Model file for the job. Use its own axes, mm. A direction names the side the tool comes from. Coordinates: 2 decimals unless noted, no trailing zeros. Write each loop counter-clockwise with the first axis right and the second up, starting at its lowest first coordinate (ties: lowest second). Pieces come first, ordered by that corner, then holes. Notation, with made-up numbers: M 60,-21 L 71,-21 A16 cw 71,-13 Z; hole C -29.5,8 d11. An arc over 180 degrees is marked long. Put each result on its own line as item: value. Start each with the question number.
Q1. Drop a flat-ended pin along its axis: pin 1 (1.5 mm diameter, centred on x = 5.5, z = -27, fed in from +Y). Give the stop position or say it passes through.
Q2. Which spindle directions (+Z, -Z, +X, -X, +Y, -Y) get a long thin tool onto all of the face, cutting with end or side? Do faces 1 (the flat face through (-2, 0, -1)), 2 (the flat face through (-2, 14.5, -27)). Say none if no direction does.
Q3. Cut at A-A (x = 2.5). Write the cut outline in (y, z).
Q4. Drill centre lines: line 1 along Z through (x, y) = (20, 15.25); line 2 along Z through (x, y) = (14, 14.75). Where is each one in solid material? Low to high.
```python
from build123d import *

# Parameters (mm, degrees)
SKETCH1_W           = 54
SKETCH1_H           = 60
BOSS_EXTRUDE1_DEPTH = 17
SKETCH2_W           = 54
SKETCH2_H           = 6
CUT_EXTRUDE1_DEPTH  = 2.5
FILLET1_R           = 1


with BuildPart() as part:
    # Sketch1 → Boss-Extrude1 (new body)
    with BuildSketch(Plane(origin=(0, 0, 0), x_dir=(1, 0, 0), z_dir=(0, 1, 0))):
        with Locations((-2.044526592, -0.229360244)):
            Rectangle(SKETCH1_W, SKETCH1_H)
    extrude(amount=BOSS_EXTRUDE1_DEPTH)

    # Sketch2 → Cut-Extrude1 (cut)
    with BuildSketch(Plane(origin=(0, 17, 0), x_dir=(1, 0, 0), z_dir=(0, 1, 0))):
        with Locations((-2.044526592, 26.770639756)):
            Rectangle(SKETCH2_W, SKETCH2_H)
    extrude(amount=-CUT_EXTRUDE1_DEPTH, mode=Mode.SUBTRACT)

    # Fillet1
    fillet1_edges = [part.edges().sort_by_distance(p)[0] for p in [
        (24.955473408, 17, 3.229360244),
        (-29.044526592, 17, 3.229360244),
        (-29.044526592, 14.5, -26.770639756),
        (-29.044526592, 15.75, -23.770639756),
        (24.955473408, 14.5, -26.770639756),
        (-2.044526592, 14.5, -23.770639756),
        (24.955473408, 15.75, -23.770639756),
        (-2.044526592, 17, -23.770639756),
        (24.955473408, 0, 0.229360244),
        (-2.044526592, 0, 30.229360244),
        (-29.044526592, 0, 0.229360244),
        (-2.044526592, 17, 30.229360244),
        (24.955473408, 8.5, 30.229360244),
        (-29.044526592, 8.5, 30.229360244),
    ]]
    fillet(fillet1_edges, radius=FILLET1_R)


solid = part.part
```
Computed values:
1. pin 1: y = 14.5
2. face 1: +Z, -Z, +X, -X, -Y
2. face 2: -Z, +X, -X, +Y
3. outline: M 0,-29.77 L 14.5,-29.77 L 14.5,-24.77 A1 cw 15.5,-23.77 L 16,-23.77 A1 ccw 17,-22.77 L 17,29.23 A1 ccw 16,30.23 L 1,30.23 A1 ccw 0,29.23 Z
4. line 1: -23.8 to 30.23
4. line 2: -24.11 to 30.23
